CAD build for the part. Positions are in the model's coordinates, mm. Face numbers are marked on the shaded views. A direction names the side the tool comes from. Give positions to 0.01 mm unless a question says otherwise; leave off trailing zeros. Loops run counter-clockwise (first coordinate to the right, second up) from the corner with the lowest first, then second, coordinate; pieces in that order, holes last. Notation, with made-up numbers: M -17,-25.75 L 13,-25.75 A24 ccw 13,5.25 Z; hole C 38,33 d7. An arc over 180 degrees is marked long. One line per question, with ' | ' between items.
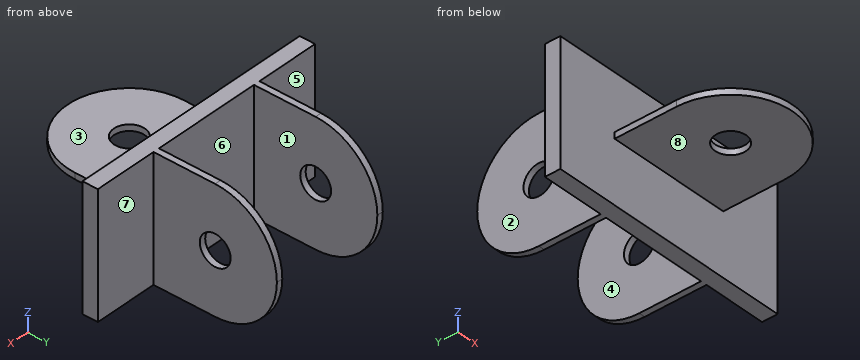
```python
from build123d import *

# Parameters (mm, degrees)
BOSS_EXTRUDE1_DEPTH = 2
SKETCH4_W           = 80
SKETCH4_H           = 5
BOSS_EXTRUDE2_DEPTH = 20
SKETCH5_W           = 2
SKETCH5_H           = 40
BOSS_EXTRUDE3_DEPTH = 40
FILLET1_R           = 20
SKETCH6_R           = 5
CUT_EXTRUDE1_DEPTH  = 80
SKETCH7_R           = 5
CUT_EXTRUDE2_DEPTH  = 80


with BuildPart() as part:
    # Sketch3 → Boss-Extrude1 (new body)
    with BuildSketch(Plane.XY):
        with BuildLine():
            Line((-20, 0), (20, 0))
            Line((20, 0), (20, -20))
            ThreePointArc((20, -20), (0, -40), (-20, -20))
            Line((-20, -20), (-20, 0))
        make_face()
    extrude(amount=BOSS_EXTRUDE1_DEPTH)

    # Sketch4 → Boss-Extrude2 (add, symmetric)
    with BuildSketch(Plane.XY):
        with Locations((0, 2.5)):
            Rectangle(SKETCH4_W, SKETCH4_H)
    extrude(amount=BOSS_EXTRUDE2_DEPTH, both=True)

    # Sketch5 → Boss-Extrude3 (add)
    with BuildSketch(Plane(origin=(0, 5, 0), x_dir=(1, 0, 0), z_dir=(0, 1, 0))):
        with Locations((-18.5, 0)):
            Rectangle(SKETCH5_W, SKETCH5_H)
        with Locations((18.5, 0)):
            Rectangle(SKETCH5_W, SKETCH5_H)
    extrude(amount=BOSS_EXTRUDE3_DEPTH)

    # Fillet1
    fillet1_edges = [part.edges().sort_by_distance(p)[0] for p in [
        (-18.5, 45, -20),
        (18.5, 45, -20),
        (-18.5, 45, 20),
        (18.5, 45, 20),
    ]]
    fillet(fillet1_edges, radius=FILLET1_R - 0.0001)  # a hair under: the kernel refuses the full size

    # Sketch6 → Cut-Extrude1 (cut)
    with BuildSketch(Plane.ZY.offset(19.5)):
        with Locations(Location((0, 25, 0), (0, 0, 270))):
            Circle(SKETCH6_R)
    extrude(amount=-CUT_EXTRUDE1_DEPTH, mode=Mode.SUBTRACT)

    # Sketch7 → Cut-Extrude2 (cut)
    with BuildSketch(Plane.XY.offset(2)):
        with Locations((0, -20)):
            Circle(SKETCH7_R)
    extrude(amount=-CUT_EXTRUDE2_DEPTH, mode=Mode.SUBTRACT)


solid = part.part
```
Item 1: Mould opens along X. For the marked faces 1, 2, 3 and 4 say: pulls with the +X half, pulls with the -X half, needs draft (parallel to the pull), parting line crosses it, or undercut.
Conclusion:
face 1: undercut | face 2: pulls with the -X half | face 3: needs draft | face 4: undercut
Item 2: Saw through at B-B on y = -23. Give the cut face in (x, z), and give its area (3 significant figures).
Conclusion:
outline: M -19.77,0 L -4,0 L -4,2 L -19.77,2 Z; M 4,0 L 19.77,0 L 19.77,2 L 4,2 Z | area: 63.1 mm²
Item 3: Saw through at A-A on x = 0. Give the cut face in (y, z), and give its area (3 significant figures).
Conclusion:
outline: M -40,0 L -25,0 L -25,2 L -40,2 Z; M -15,0 L 0,0 L 0,-20 L 5,-20 L 5,20 L 0,20 L 0,2 L -15,2 Z | area: 260 mm²
Item 4: Drop flat-ended pins along their axis: P1, Ø2, axis at y = 34.5, z = 7.5, coming from the -X side; P2, Ø3, axis at x = -9, y = -22, coming from the -Z side; P3, Ø8, axis at x = -25.5, z = -5.5, coming from the -Y side. Give the stop position or say it passes through.
Conclusion:
P1: x = -19.5 | P2: z = 0 | P3: y = 0
Item 5: Drill centre lines: line 1 along X through (y, z) = (41.5, 2.5); line 2 along Y through (x, z) = (0, 1); line 3 along Z through (x, y) = (18, 25). Where is each one in solid material? Low to high. Write a range as [from, to].
Conclusion:
line 1: [-19.5, -17.5], [17.5, 19.5] | line 2: [-40, -25], [-15, 5] | line 3: [-20, -5], [5, 20]
Item 6: 3-axis set-ups, long thin cutter, end or side, ignore diameter. For the marked faces 5, 6, 7 and 8: which of +Z, -Z, +X, -X, +Y, -Y reach the whole face in a straight line?
Conclusion:
face 5: +Z, -Z, -X, +Y | face 6: +Z, -Z, +Y | face 7: +Z, -Z, +X, +Y | face 8: -Z, +X, -X, -Y
Item 7: Saw through at C-C on z = 4. Give the cut face in (x, y).
Conclusion:
outline: M -40,0 L 40,0 L 40,5 L 19.5,5 L 19.5,22 L 17.5,22 L 17.5,5 L -17.5,5 L -17.5,22 L -19.5,22 L -19.5,5 L -40,5 Z; M -19.5,28 L -17.5,28 L -17.5,44.6 L -19.5,44.6 Z; M 17.5,28 L 19.5,28 L 19.5,44.6 L 17.5,44.6 Z
Item 8: Saw through at D-D on z = 9.5. Give the cut face in (x, y).
Conclusion:
outline: M -40,0 L 40,0 L 40,5 L 19.5,5 L 19.5,42.6 L 17.5,42.6 L 17.5,5 L -17.5,5 L -17.5,42.6 L -19.5,42.6 L -19.5,5 L -40,5 Z
